```python
from build123d import *

# Parameters (mm, degrees)
SKETCH1_R           = 7.5
SKETCH1_R_2         = 3
BOSS_EXTRUDE1_DEPTH = 19.8
CUT_EXTRUDE1_START  = 3.9
SKETCH1_6_R         = 7.5
SKETCH1_6_R_2       = 3
CUT_EXTRUDE1_DEPTH  = 12
SKETCH1_7_R         = 7.5
SKETCH1_7_R_2       = 3
CUT_EXTRUDE5_DEPTH  = 20.8


with BuildPart() as part:
    # Sketch1 → Boss-Extrude1 (new body)
    with BuildSketch(Plane.XY):
        Circle(SKETCH1_R)
        Circle(SKETCH1_R_2, mode=Mode.SUBTRACT)
        Circle(SKETCH1_R_2)
    extrude(amount=BOSS_EXTRUDE1_DEPTH)

    # Sketch1_6 → Cut-Extrude1 (cut)
    with BuildSketch(Plane.XY.offset(CUT_EXTRUDE1_START)):
        Circle(SKETCH1_6_R)
        Circle(SKETCH1_6_R_2, mode=Mode.SUBTRACT)
    extrude(amount=CUT_EXTRUDE1_DEPTH, mode=Mode.SUBTRACT)

    # Sketch1_7 → Cut-Extrude5 (cut, through all)
    with BuildSketch(Plane.XY):
        Circle(SKETCH1_7_R)
        Circle(SKETCH1_7_R_2, mode=Mode.SUBTRACT)
    extrude(amount=CUT_EXTRUDE5_DEPTH, mode=Mode.SUBTRACT)


solid = part.part
```
The model under review builds one solid part; all positions refer to its coordinate system, in mm. Round coordinates to 2 decimals unless told otherwise and drop trailing zeros. Loops run counter-clockwise (first coordinate to the right, second up) from the corner with the lowest first, then second, coordinate; pieces in that order, holes last. Notation, with made-up numbers: (5, 10) - (11, 10) arc R20 cw to (11, 24) - close; hole circle Ø5 at (56.25, 23.25). An arc over 180 degrees is marked (long way). Use a Markdown table: item, result. Add a question column.
Q1. Add section B-B (x = 1.8). State the section outline as (y, z) points, plus the area to 3 significant figures.
Q2. Add section A-A (z = 18.5). State the section outline as (x, y) points.
Q3. Add section C-C (y = 2.45). State the section outline as (x, z) points.
Q4. For probe 1 along Y at (x, z) = (-0.15, 6.25); probe 2 along X at (y, z) = (0.85, 6.25); probe 3 along Y at (x, z) = (-1.95, 18), list the stretches that pass through material, from the lowest coordinate up.
Q5. Insertion check: pin 1 Ø1.5 at (x, y) = (0, -0.5) entering from -Z; pin 2 Ø3 at (y, z) = (-2, 9.5) entering from -X; pin 3 Ø1 at (y, z) = (1.5, 4) entering from +X. Each pin has a flat end and moves straight along its axis. Give the tip position at first contact, or say it passes through.
Worked answers:
| question | item | result |
|---|---|---|
| 1 | outline | (-2.4, 0) - (2.4, 0) - (2.4, 19.8) - (-2.4, 19.8) - close |
| 1 | area | 95.0 mm² |
| 2 | outline | circle Ø6 at (0, 0) |
| 3 | outline | (-1.73, 0) - (1.73, 0) - (1.73, 19.8) - (-1.73, 19.8) - close |
| 4 | probe 1 | -3 to 3 |
| 4 | probe 2 | -2.88 to 2.88 |
| 4 | probe 3 | -2.28 to 2.28 |
| 5 | pin 1 | z = 0 |
| 5 | pin 2 | x = -2.96 |
| 5 | pin 3 | x = 2.83 |
